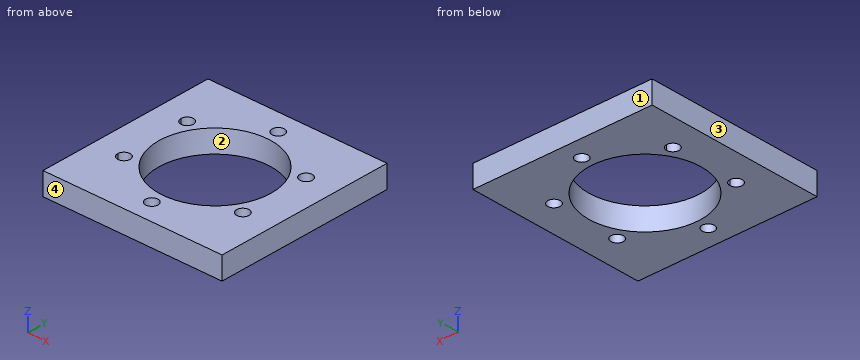
from build123d import *

# Parameters (mm, degrees)
SKETCH1_W           = 50.8
SKETCH1_H           = 50.8
SKETCH1_R           = 15.875
BOSS_EXTRUDE1_DEPTH = 6.35


with BuildPart() as part:
    # Sketch1 → Boss-Extrude1 (new body)
    with BuildSketch(Plane.XY):
        with Locations((19.355037388, 24.095046544)):
            Rectangle(SKETCH1_W, SKETCH1_H)
        with Locations((19.355037388, 24.095046544)):
            Circle(SKETCH1_R, mode=Mode.SUBTRACT)
        with BuildLine():
            ThreePointArc((34.45579594, 14.360477203), (36.215806077, 12.600467066), (37.975816214, 14.360477203))
            ThreePointArc((37.975816214, 14.360477203), (36.215806077, 16.12048734), (34.45579594, 14.360477203))
        make_face(mode=Mode.SUBTRACT)
        with BuildLine():
            ThreePointArc((21.115047525, 4.625907862), (19.355037388, 6.385917999), (17.595027251, 4.625907862))
            ThreePointArc((17.595027251, 4.625907862), (19.355037388, 2.865897725), (21.115047525, 4.625907862))
        make_face(mode=Mode.SUBTRACT)
        with BuildLine():
            ThreePointArc((17.595027251, 43.564185227), (19.355037388, 41.80417509), (21.115047525, 43.564185227))
            ThreePointArc((21.115047525, 43.564185227), (19.355037388, 45.324195364), (17.595027251, 43.564185227))
        make_face(mode=Mode.SUBTRACT)
        with BuildLine():
            ThreePointArc((37.975816214, 33.829615886), (36.215806077, 35.589626023), (34.45579594, 33.829615886))
            ThreePointArc((34.45579594, 33.829615886), (36.215806077, 32.069605749), (37.975816214, 33.829615886))
        make_face(mode=Mode.SUBTRACT)
        with BuildLine():
            ThreePointArc((0.734258563, 33.829615886), (2.494268699, 32.069605749), (4.254278836, 33.829615886))
            ThreePointArc((4.254278836, 33.829615886), (2.494268699, 35.589626023), (0.734258563, 33.829615886))
        make_face(mode=Mode.SUBTRACT)
        with BuildLine():
            ThreePointArc((4.254278836, 14.360477203), (2.494268699, 16.12048734), (0.734258563, 14.360477203))
            ThreePointArc((0.734258563, 14.360477203), (2.494268699, 12.600467066), (4.254278836, 14.360477203))
        make_face(mode=Mode.SUBTRACT)
    extrude(amount=BOSS_EXTRUDE1_DEPTH)


solid = part.part
Read the model definition and answer for the solid it produces. Units are mm, in the model's axes. Face numbers are marked on the shaded views. Round coordinates to 2 decimals unless told otherwise and drop trailing zeros. Write each loop counter-clockwise with the first axis right and the second up, starting at its lowest first coordinate (ties: lowest second). Pieces come first, ordered by that corner, then holes. Notation, with made-up numbers: (74, 33) - (97, 33) arc R26 cw to (97, 47) - close; hole circle Ø2 at (0, -14.5). An arc over 180 degrees is marked (long way). One line per question, with ' | ' between items. Start each with the question number.
1. For a pull along Y with two mould halves and no side action, classify the marked faces 1, 2, 3 and 4 as +Y half, -Y half, draft (parallel to the pull), parting line (faces both ways), or undercut.
2. Section B-B (y = 39) is taken. Determine the outline of the cut face in (x, z).
3. This flat-tipped pin is pushed along its axis until it touches: pin 1 (2 mm diameter, centred on x = 19.36, y = 43.56, fed in from -Z). Where does it stop, or does it pass through?
4. Section C-C (x = 37) is taken. Determine the outline of the cut face in (y, z).
5. Section D-D (z = 2) is taken. Determine the outline of the cut face in (x, y) (3 decimals).
6. Find the intervals of material crossed by probe 1 along X at (y, z) = (29, 6); probe 2 along X at (y, z) = (14.5, 1.25); probe 3 along X at (y, z) = (15, 3.25), in increasing order. Write a range as [from, to].
7. Section A-A (x = 14.5) is taken. Determine the outline of the cut face in (y, z), and give its area (3 significant figures).
Filled in:
1) face 1: +Y half | face 2: undercut | face 3: draft | face 4: -Y half
2) outline: (-6.04, 0) - (13.89, 0) - (13.89, 6.35) - (-6.04, 6.35) - close; (24.82, 0) - (44.76, 0) - (44.76, 6.35) - (24.82, 6.35) - close
3) pin 1: through
4) outline: (-1.3, 0) - (12.78, 0) - (12.78, 6.35) - (-1.3, 6.35) - close; (15.94, 0) - (32.25, 0) - (32.25, 6.35) - (15.94, 6.35) - close; (35.41, 0) - (49.5, 0) - (49.5, 6.35) - (35.41, 6.35) - close
5) outline: (-6.045, -1.305) - (44.755, -1.305) - (44.755, 49.495) - (-6.045, 49.495) - close; hole circle Ø3.52 at (2.494, 14.36); hole circle Ø3.52 at (2.494, 33.83); hole circle Ø31.75 at (19.355, 24.095); hole circle Ø3.52 at (19.355, 4.626); hole circle Ø3.52 at (19.355, 43.564); hole circle Ø3.52 at (36.216, 14.36); hole circle Ø3.52 at (36.216, 33.83)
6) probe 1: [-6.04, 4.26], [34.45, 44.76] | probe 2: [-6.04, 0.74], [4.25, 6.71], [32, 34.46], [37.97, 44.76] | probe 3: [-6.04, 0.85], [4.13, 6.34], [32.37, 34.58], [37.86, 44.76]
7) outline: (-1.3, 0) - (8.98, 0) - (8.98, 6.35) - (-1.3, 6.35) - close; (39.21, 0) - (49.5, 0) - (49.5, 6.35) - (39.21, 6.35) - close | area: 131 mm²
